Read the model definition and answer for the solid it produces. Units are mm, in the model's axes. Face numbers are marked on the shaded views. A direction names the side the tool comes from. Coordinates: 2 decimals unless noted, no trailing zeros. Order: outer loops, then holes, each group sorted by start corner. A loop starts at its lowest first (then second) coordinate and runs counter-clockwise, first axis right, second up. Notation, with made-up numbers: (-11, -32) -> (5, -32) arc R24 cw to (5, -9) -> close; hole circle Ø10 at (-17.75, 37.5). An arc over 180 degrees is marked (long way). Answer in a Markdown table with one row per item.
from build123d import *

# Parameters (mm, degrees)
SKETCH_1_W      = 40
SKETCH_1_H      = 22
EXTRUDE_1_DEPTH = 9
SKETCH_2_W      = 8
SKETCH_2_H      = 22
EXTRUDE_2_DEPTH = 5


with BuildPart() as part:
    # Эскиз1 → Бобышка-Вытянуть1 (new body)
    with BuildSketch(Plane(origin=(0, 0, 0), x_dir=(1, 0, 0), z_dir=(0, 1, 0))):
        Rectangle(SKETCH_1_W, SKETCH_1_H)
    extrude(amount=EXTRUDE_1_DEPTH)

    # Эскиз2 → Бобышка-Вытянуть2 (add)
    with BuildSketch(Plane(origin=(0, 9, 0), x_dir=(1, 0, 0), z_dir=(0, 1, 0))):
        with Locations((16, 0)):
            Rectangle(SKETCH_2_W, SKETCH_2_H)
    extrude(amount=EXTRUDE_2_DEPTH)


solid = part.part
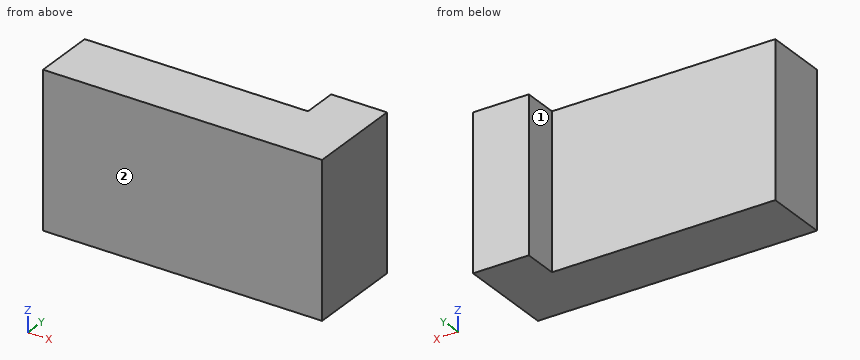
Q1. The part is cut by section A-A (z = 1.25). Write down the section's boundary in (x, y).
Outcome:
| item | result |
|---|---|
| outline | (-20, 0) -> (20, 0) -> (20, 14) -> (12, 14) -> (12, 9) -> (-20, 9) -> close |
Q2. The part is cut by section C-C (x = -11). Write down the section's boundary in (y, z), then the cut area to 3 significant figures.
Outcome:
| item | result |
|---|---|
| outline | (0, -11) -> (9, -11) -> (9, 11) -> (0, 11) -> close |
| area | 198 mm² |
Q3. Given pin 1 (6.5 mm diameter, centred on x = -7, z = -1, fed in from +Y); pin 2 (1.5 mm diameter, centred on y = 10.5, z = 1.5, fed in from -X), each flat-ended and moving along its own axis, determine where each tip first touches the part or whether it passes through.
Outcome:
| item | result |
|---|---|
| pin 1 | y = 9 |
| pin 2 | x = 12 |
Q4. For the marked faces 1 and 2, determine the directions among +Z, -Z, +X, -X, +Y, -Y from which every point of the face is accessible in a straight line to the end or side of a thin tool.
Outcome:
| item | result |
|---|---|
| face 1 | +Z, -Z, -X, +Y |
| face 2 | +Z, -Z, +X, -X, -Y |
Q5. Consider line 1 (X direction, y = 9.25, z = 4.5); line 2 (Y direction, x = 8, z = -6.25). Determine where each line is inside the solid, lowest interval first.
Outcome:
| item | result |
|---|---|
| line 1 | 12 to 20 |
| line 2 | 0 to 9 |
Q6. The part is cut by section B-B (y = 13.25). Write down the section's boundary in (x, z).
Outcome:
| item | result |
|---|---|
| outline | (12, -11) -> (20, -11) -> (20, 11) -> (12, 11) -> close |
